```python
from build123d import *

# Parameters (mm, degrees)
F0_W           = 118
F0_H           = 75
F0_R           = 2.75
F0_R_2         = 1.6
F0_W_2         = 14
F0_H_2         = 20
F1_DEPTH       = 8
F3_D           = 5.5
F3_DEPTH       = 8
F3_CBORE_D     = 9.75
F3_CBORE_DEPTH = 5
F4_D           = 3.4
F4_DEPTH       = 8
F4_CBORE_D     = 5.4
F4_CBORE_DEPTH = 4


with BuildPart() as f1:
    # F0 (on Top) → F1 (new body)
    with BuildSketch(Plane.XY):
        Rectangle(F0_W, F0_H)
        with Locations((-49, -21.5)):
            Circle(F0_R, mode=Mode.SUBTRACT)
        with Locations((39, -33.5)):
            Circle(F0_R_2, mode=Mode.SUBTRACT)
        with Locations((46, -33.5)):
            Circle(F0_R_2, mode=Mode.SUBTRACT)
        with Locations((51, -21.5)):
            Circle(F0_R, mode=Mode.SUBTRACT)
        with Locations((-49, 13.5)):
            Circle(F0_R, mode=Mode.SUBTRACT)
        with Locations((-34, 14.5)):
            Rectangle(F0_W_2, F0_H_2, mode=Mode.SUBTRACT)
        with Locations((11, 22.5)):
            Circle(F0_R, mode=Mode.SUBTRACT)
        with Locations((39, 33.5)):
            Circle(F0_R_2, mode=Mode.SUBTRACT)
        with Locations((46, 33.5)):
            Circle(F0_R_2, mode=Mode.SUBTRACT)
    extrude(amount=F1_DEPTH)

    # F3
    with Locations(Plane.XY.offset(8)):
        with Locations((-49, 13.5), (11, 22.5), (51, -21.5), (-49, -21.5)):
            CounterBoreHole(F3_D / 2, F3_CBORE_D / 2, F3_CBORE_DEPTH, depth=F3_DEPTH)

    # F4
    with Locations(Plane.XY.offset(8)):
        with Locations((39, -33.5), (46, -33.5), (39, 33.5), (46, 33.5)):
            CounterBoreHole(F4_D / 2, F4_CBORE_D / 2, F4_CBORE_DEPTH, depth=F4_DEPTH)


solid = f1.part
```
Work out the finished part from the listing and answer in its coordinate system (mm). A direction names the side the tool comes from. Give positions to 0.01 mm unless a question says otherwise; leave off trailing zeros. Write each loop counter-clockwise with the first axis right and the second up, starting at its lowest first coordinate (ties: lowest second). Pieces come first, ordered by that corner, then holes. Notation, with made-up numbers: (-31, 41.5) - (-27, 41.5) arc R7 ccw to (-27, 54.5) - close; hole circle Ø9 at (19.5, 69.5). An arc over 180 degrees is marked (long way). Use one line per item in the form item = value.
1. A cutting plane is placed at C-C (z = 5.5). State how many separate pieces and enclosed holes the cut face has, and give its area (3 significant figures).
Filled in:
separate_pieces = 1
enclosed_holes = 9
area = 8,180 mm^2
2. Each of these flat-tipped pins is pushed along its axis until it touches: pin 1 Ø2.5 at (x, y) = (39.5, 34.5) entering from +Z; pin 2 Ø5 at (x, y) = (-49.5, -23) entering from +Z; pin 3 Ø2.5 at (x, y) = (46, 33.5) entering from -Z (1 decimal). Where does it stop, or does it pass through?
Filled in:
pin_1 = 4
pin_2 = 3
pin_3 = through
3. A cutting plane is placed at B-B (y = -33.5). Write down the section's boundary in (x, z).
Filled in:
outline = (-59, 0) - (37.3, 0) - (37.3, 4) - (36.3, 4) - (36.3, 8) - (-59, 8) - close; (40.7, 0) - (44.3, 0) - (44.3, 4) - (43.3, 4) - (43.3, 8) - (41.7, 8) - (41.7, 4) - (40.7, 4) - close; (47.7, 0) - (59, 0) - (59, 8) - (48.7, 8) - (48.7, 4) - (47.7, 4) - close
4. Consider L1, parallel to Y at x = -49, z = 1.5; L2, parallel to Y at x = 39, z = 5.1; L3, parallel to X at y = -23, z = 7. Determine where each line is inside the solid, lowest interval first.
Filled in:
L1 = -37.5 to -24.25, -18.75 to 10.75, 16.25 to 37.5
L2 = -37.5 to -36.2, -30.8 to 30.8, 36.2 to 37.5
L3 = -59 to -53.64, -44.36 to 46.36, 55.64 to 59
5. Determine the mould class of faces 1 (the face through (-1, 37.5, 4)), 2 (the face through (59, -1, 4)), 3 (the face through (41.575, -32.689, 6.028)) for opening direction X: released by +X, released by -X, zero draft, split by the parting line, or undercut.
Filled in:
face_1 = zero draft
face_2 = released by +X
face_3 = undercut
6. A cutting plane is placed at D-D (x = 11). Write down the section's boundary in (y, z) (3 decimals), and give its area (3 significant figures).
Filled in:
outline = (-37.5, 0) - (19.75, 0) - (19.75, 3) - (17.625, 3) - (17.625, 8) - (-37.5, 8) - close; (25.25, 0) - (37.5, 0) - (37.5, 8) - (27.375, 8) - (27.375, 3) - (25.25, 3) - close
area = 535 mm^2
7. For faces 4 (the face through (-51.747, -21.379, 1.479)), 5 (the face through (41.575, 34.311, 6.028)), determine the directions among +Z, -Z, +X, -X, +Y, -Y from which every point of the face is accessible in a straight line to the end or side of a thin tool.
Filled in:
face_4 = +Z, -Z
face_5 = +Z
8. A cutting plane is placed at A-A (x = -49). Write down the section's boundary in (y, z) (3 decimals).
Filled in:
outline = (-37.5, 0) - (-24.25, 0) - (-24.25, 3) - (-26.375, 3) - (-26.375, 8) - (-37.5, 8) - close; (-18.75, 0) - (10.75, 0) - (10.75, 3) - (8.625, 3) - (8.625, 8) - (-16.625, 8) - (-16.625, 3) - (-18.75, 3) - close; (16.25, 0) - (37.5, 0) - (37.5, 8) - (18.375, 8) - (18.375, 3) - (16.25, 3) - close
